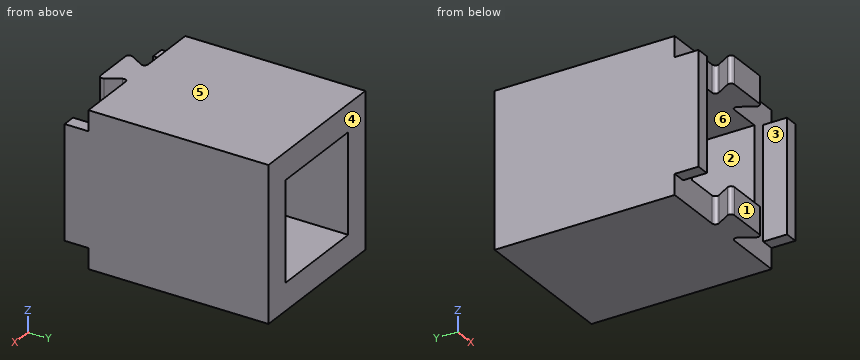
```python
from build123d import *

# Parameters (mm, degrees)
SKETCH1_W           = 22.6
SKETCH1_H           = 22.6
SKETCH1_W_2         = 14.6
SKETCH1_H_2         = 14.6
BOSS_EXTRUDE1_DEPTH = 30
CUT_EXTRUDE1_DEPTH  = 40.22307994
FILLET1_R           = 0.5
SKETCH3_W           = 1.95
SKETCH3_H           = 16.6
BOSS_EXTRUDE2_DEPTH = 3.5


with BuildPart() as part:
    # Sketch1 → Boss-Extrude1 (new body)
    with BuildSketch(Plane(origin=(0, 0, 0), x_dir=(1, 0, 0), z_dir=(0, 1, 0))):
        Rectangle(SKETCH1_W, SKETCH1_H)
        Rectangle(SKETCH1_W_2, SKETCH1_H_2, mode=Mode.SUBTRACT)
    extrude(amount=BOSS_EXTRUDE1_DEPTH)

    # Sketch2 → Cut-Extrude1 (cut, through all)
    with BuildSketch(Plane.XY.offset(11.3)):
        Polygon((3.770725942, 0), (1.75, 3.5), (11.3, 3.5), (11.3, 0), align=None)
        Polygon((-11.3, 3.5), (-11.3, 0), (-3.770725942, 0), (-1.75, 3.5), align=None)
    extrude(amount=-CUT_EXTRUDE1_DEPTH, mode=Mode.SUBTRACT)

    # Fillet1
    fillet1_edges = [part.edges().sort_by_distance(p)[0] for p in [
        (3.770725942, 0, -9.3),
        (3.770725942, 0, 9.3),
        (1.75, 3.5, 9.3),
        (1.75, 3.5, -9.3),
        (-1.75, 3.5, -9.3),
        (-1.75, 3.5, 9.3),
        (-3.770725942, 0, 9.3),
        (-3.770725942, 0, -9.3),
    ]]
    fillet(fillet1_edges, radius=FILLET1_R)

    # Sketch3 → Boss-Extrude2 (add)
    with BuildSketch(Plane(origin=(0, 3.5, 0), x_dir=(-1, 0, 0), z_dir=(0, -1, 0))):
        with Locations((-10.325, 0)):
            Rectangle(SKETCH3_W, SKETCH3_H)
        with Locations((10.325, 0)):
            Rectangle(SKETCH3_W, SKETCH3_H)
    extrude(amount=BOSS_EXTRUDE2_DEPTH)


solid = part.part
```
Can you work these out from the model? Positions are in its coordinate system, mm. Face numbers are marked on the shaded views. A direction names the side the tool comes from. Coordinates: 2 decimals unless noted, no trailing zeros. Loops run counter-clockwise (first coordinate to the right, second up) from the corner with the lowest first, then second, coordinate; pieces in that order, holes last.
1) Imagine slicing it at D-D on x = 1. List the corners of the cut face in (y, z) for me.
2) Imagine slicing it at B-B on z = 5.75. List the corners of the cut face in (x, y) for me.
3) For pin 1 (1.6 mm diameter, centred on x = -10.5, y = 1, fed in from +Z); pin 2 (1 mm diameter, centred on x = -10.5, y = 1, fed in from -Z); pin 3 (4 mm diameter, centred on x = -3.5, z = 6.5, fed in from -Y); pin 4 (4 mm diameter, centred on x = 3, z = 4.5, fed in from -Y), each with a flat end and sliding along its axis, tell me the tip position at first contact or that it passes through.
4) Thinking about a two-plate mould opening in Z: for the marked faces 4, 5 and 6, which applies, pulls with the +Z half, pulls with the -Z half, needs draft (parallel to the pull), parting line crosses it, or undercut?
5) Which directions (+Z, -Z, +X, -X, +Y, -Y) give clear straight access to the entire face, cutting with the end or side of a thin tool? Please do the marked faces 1, 2 and 3.
6) Imagine slicing it at A-A on x = 4.75. List the corners of the cut face in (y, z) for me.
7) I need wall thicknesses on probe 1 along Z at (x, y) = (5, 7.25); probe 2 along Y at (x, z) = (-6.5, -7.5). Which ranges of each line are inside material? Lowest first, please.
8) Imagine slicing it at C-C on y = 4.75. List the corners of the cut face in (x, z) for me, plus the area to 3 significant figures.
Completed:
1. outline: (0, -11.3) - (30, -11.3) - (30, -7.3) - (0, -7.3) - close; (0, 7.3) - (30, 7.3) - (30, 11.3) - (0, 11.3) - close
2. outline: (-11.3, 0) - (-9.35, 0) - (-9.35, 3.5) - (-7.3, 3.5) - (-7.3, 30) - (-11.3, 30) - close; (7.3, 3.5) - (9.35, 3.5) - (9.35, 0) - (11.3, 0) - (11.3, 30) - (7.3, 30) - close
3. pin 1: stops at z = 8.3
3. pin 2: stops at z = -8.3
3. pin 3: stops at y = 0
3. pin 4: passes through
4. face 4: needs draft
4. face 5: pulls with the +Z half
4. face 6: undercut
5. face 1: +Z, -Z, +X, -X, -Y
5. face 2: +Y, -Y
5. face 3: +Z, -Z, -Y
6. outline: (3.5, -11.3) - (30, -11.3) - (30, -7.3) - (3.5, -7.3) - close; (3.5, 7.3) - (30, 7.3) - (30, 11.3) - (3.5, 11.3) - close
7. probe 1: z = -11.3 to -7.3, 7.3 to 11.3
7. probe 2: y = 3.5 to 30
8. outline: (-11.3, -11.3) - (11.3, -11.3) - (11.3, 11.3) - (-11.3, 11.3) - close; hole (-7.3, -7.3) - (7.3, -7.3) - (7.3, 7.3) - (-7.3, 7.3) - close
8. area: 298 mm2
